from build123d import *

# Parameters (mm, degrees)
ESQUISSE1_W              = 305
ESQUISSE1_H              = 305
BOSS_EXTRU_1_DEPTH       = 10
ESQUISSE2_R              = 10
ENL_V_MAT_EXTRU_10_DEPTH = 10
CONG_2_R                 = 15
ESQUISSE3_R              = 5
ENL_V_MAT_EXTRU_11_DEPTH = 10
ESQUISSE4_R              = 15
BOSS_EXTRU_2_DEPTH       = 10
ESQUISSE5_R              = 7.5
ENL_V_MAT_EXTRU_12_DEPTH = 20
ESQUISSE6_R              = 5
ENL_V_MAT_EXTRU_13_DEPTH = 10


with BuildPart() as part:
    # Esquisse1 → Boss.-Extru.1 (new body)
    with BuildSketch(Plane.XY):
        Rectangle(ESQUISSE1_W, ESQUISSE1_H)
    extrude(amount=BOSS_EXTRU_1_DEPTH)

    # Esquisse2 → Enlèv. mat.-Extru.10 (cut)
    with BuildSketch(Plane.XY.offset(10)):
        with Locations((137.5, 137.5)):
            Circle(ESQUISSE2_R)
        with Locations((137.5, -137.5)):
            Circle(ESQUISSE2_R)
        with Locations((-137.5, -137.5)):
            Circle(ESQUISSE2_R)
        with Locations((-137.5, 137.5)):
            Circle(ESQUISSE2_R)
    extrude(amount=-ENL_V_MAT_EXTRU_10_DEPTH, mode=Mode.SUBTRACT)

    # Congé2
    cong_2_edges = [part.edges().sort_by_distance(p)[0] for p in [
        (-152.5, 152.5, 5),
        (152.5, 152.5, 5),
        (152.5, -152.5, 5),
        (-152.5, -152.5, 5),
    ]]
    fillet(cong_2_edges, radius=CONG_2_R)

    # Esquisse3 → Enlèv. mat.-Extru.11 (cut)
    with BuildSketch(Plane.XY.offset(10)):
        with Locations((80, 80)):
            Circle(ESQUISSE3_R)
        with Locations((80, -80)):
            Circle(ESQUISSE3_R)
        with Locations((-80, -80)):
            Circle(ESQUISSE3_R)
        with Locations((-80, 80)):
            Circle(ESQUISSE3_R)
    extrude(amount=-ENL_V_MAT_EXTRU_11_DEPTH, mode=Mode.SUBTRACT)

    # Esquisse4 → Boss.-Extru.2 (add)
    with BuildSketch(Plane.XY.offset(10)):
        with Locations(Location((0, 0, 0), (0, 0, 180))):
            Circle(ESQUISSE4_R)
    extrude(amount=BOSS_EXTRU_2_DEPTH)

    # Esquisse5 → Enlèv. mat.-Extru.12 (cut)
    with BuildSketch(Plane.XY.offset(20)):
        Circle(ESQUISSE5_R)
    extrude(amount=-ENL_V_MAT_EXTRU_12_DEPTH, mode=Mode.SUBTRACT)

    # Esquisse6 → Enlèv. mat.-Extru.13 (cut)
    with BuildSketch(Plane.XY.offset(10)):
        with Locations((0, 25)):
            Circle(ESQUISSE6_R)
        with Locations((0, -25)):
            Circle(ESQUISSE6_R)
    extrude(amount=-ENL_V_MAT_EXTRU_13_DEPTH, mode=Mode.SUBTRACT)


solid = part.part
Part model, mm, in its own coordinate system. A direction names the side the tool comes from. Coordinates: 2 decimals unless noted, no trailing zeros. Write each loop counter-clockwise with the first axis right and the second up, starting at its lowest first coordinate (ties: lowest second). Pieces come first, ordered by that corner, then holes. Notation, with made-up numbers: (-30.5, 78.25) - (14.5, 78.25) arc R18 cw to (14.5, 88.25) - close; hole circle Ø8 at (-17, 75). An arc over 180 degrees is marked (long way). Put each result on its own line as item: value.
1. Band-saw the part on B-B (x = 0). Write the cut outline in (y, z).
Final values:
outline: (-152.5, 0) - (-30, 0) - (-30, 10) - (-152.5, 10) - close; (-20, 0) - (-7.5, 0) - (-7.5, 20) - (-15, 20) - (-15, 10) - (-20, 10) - close; (7.5, 0) - (20, 0) - (20, 10) - (15, 10) - (15, 20) - (7.5, 20) - close; (30, 0) - (152.5, 0) - (152.5, 10) - (30, 10) - close
2. Band-saw the part on A-A (x = 80). Write the cut outline in (y, z).
Final values:
outline: (-152.5, 0) - (-85, 0) - (-85, 10) - (-152.5, 10) - close; (-75, 0) - (75, 0) - (75, 10) - (-75, 10) - close; (85, 0) - (152.5, 0) - (152.5, 10) - (85, 10) - close
3. Two-plate mould, pull along X, no slides. Class faces 1 (the cylindrical face through (84.619, -81.915, 5.07)), 2 (the cylindrical face through (-148.22, -147.99, 5.07)), 3 (the flat face through (-2, 152.5, 5)): +X half, -X half, draft (parallel to the pull), parting line (faces both ways), or undercut.
Final values:
face 1: undercut
face 2: -X half
face 3: draft
4. Band-saw the part on D-D (y = 69.5). Write the cut outline in (x, z), then the cut area to 3 significant figures.
Final values:
outline: (-152.5, 0) - (152.5, 0) - (152.5, 10) - (-152.5, 10) - close
area: 3,050 mm²
5. Probe line 1 along Y through (x, z) = (0, 5.25); line 2 along Y through (x, z) = (-137.5, 5.25); line 3 along X through (y, z) = (-76, 8.5). List the from-to ranges inside material, lowest first. Write a range as [from, to].
Final values:
line 1: y = [-152.5, -30], [-20, -7.5], [7.5, 20], [30, 152.5]
line 2: y = [-152.5, -147.5], [-127.5, 127.5], [147.5, 152.5]
line 3: x = [-152.5, -83], [-77, 77], [83, 152.5]
6. 3-axis set-ups, long thin cutter, end or side, ignore diameter. For faces 4 (the cylindrical face through (-1.08, -29.88, 5.07)), 5 (the cylindrical face through (-8.06, -12.65, 14.93)): which of +Z, -Z, +X, -X, +Y, -Y reach the whole face in a straight line?
Final values:
face 4: +Z, -Z
face 5: +Z
7. Flat gauge pins, fed straight in: pin 1 Ø4 at (x, y) = (81.5, 57.5) entering from -Z; pin 2 Ø11.5 at (x, y) = (0, -25) entering from +Z; pin 3 Ø16 at (x, y) = (-137.5, -137.5) entering from +Z. Where does each tip first touch, or does it go through?
Final values:
pin 1: stops at z = 0
pin 2: stops at z = 10
pin 3: passes through
